Check sheet for the modelled part. Datum: model origin and axes. Units: mm. A direction names the side the tool comes from. Give positions to 0.01 mm unless a question says otherwise; leave off trailing zeros. Order: outer loops, then holes, each group sorted by start corner. A loop starts at its lowest first (then second) coordinate and runs counter-clockwise, first axis right, second up. Notation, with made-up numbers: (55.5, 34.5) - (95.5, 34.5) arc R29 cw to (95.5, 64.5) - close; hole circle Ø3 at (-30.5, 24.5). An arc over 180 degrees is marked (long way). Answer in a Markdown table with one row per item.
from build123d import *

# Parameters (mm, degrees)
F0_R     = 2.55
F1_DEPTH = 100
F2_R     = 2.75
F3_DEPTH = 15
F4_R     = 3


with BuildPart() as f1:
    # F0 (on Right) → F1 (new body)
    with BuildSketch(Plane.YZ):
        with BuildLine():
            Line((0, 57.5), (0, 0))
            Line((0, 0), (55, 0))
            Line((55, 0), (55, 15))
            Line((55, 15), (33, 15))
            ThreePointArc((33, 15), (27.343146, 17.343146), (25, 23))
            Line((25, 23), (25, 57.5))
            Line((25, 57.5), (0, 57.5))
        make_face()
        with Locations((12.5, 45)):
            Circle(F0_R, mode=Mode.SUBTRACT)
    extrude(amount=F1_DEPTH)

    # F2 (on Top) → F3 (cut)
    with BuildSketch(Plane.XY):
        with Locations((15, 45)):
            Circle(F2_R)
        with Locations((85, 45)):
            Circle(F2_R)
    extrude(amount=F3_DEPTH, mode=Mode.SUBTRACT)

    # F4
    f4_edges = [f1.edges().sort_by_distance(p)[0] for p in [
        (100, 12.5, 57.5),
        (0, 12.5, 57.5),
        (50, 25, 57.5),
        (50, 0, 57.5),
        (100, 44, 15),
        (50, 55, 15),
        (0, 44, 15),
        (100, 0, 28.75),
        (0, 0, 28.75),
        (0, 55, 7.5),
        (100, 55, 7.5),
    ]]
    fillet(f4_edges, radius=F4_R)


solid = f1.part
(1) Mould release check, pull along Z, two halves, no side actions. Record for faces 1 (the cylindrical face through (49.342, 27.406, 17.281)), 2 (the cylindrical face through (49.3, 10.6, 46.7)), 3 (the flat face through (49, 27, 0)): pulls with the +Z half, pulls with the -Z half, needs draft (parallel to the pull), parting line crosses it, or undercut.
Geometry says:
| item | result |
|---|---|
| face 1 | pulls with the +Z half |
| face 2 | undercut |
| face 3 | pulls with the -Z half |
(2) Access from +Z, -Z, +X, -X, +Y, -Y to the whole of each face (thin tool, end or side, straight path). Record for faces 4 (the cylindrical face through (0.86, 42.37, 14.1)), 5 (the flat face through (49, 43, 15)), 6 (the cylindrical face through (99.1, 0.86, 26.87)).
Geometry says:
| item | result |
|---|---|
| face 4 | +Z, -X, +Y |
| face 5 | +Z, +X, -X, +Y |
| face 6 | +Z, -Z, +X, -Y |
(3) Thickness scan on L1, parallel to Y at x = 85, z = 9.5; L2, parallel to Z at x = 58, y = 40.5; L3, parallel to Z at x = 34, y = 12.5. Record the ranges inside material, lowest first.
Geometry says:
| item | result |
|---|---|
| L1 | 0 to 42.25, 47.75 to 55 |
| L2 | 0 to 15 |
| L3 | 0 to 42.45, 47.55 to 57.5 |
(4) Cross-section at B-B, the plane x = 15. Record the cut outline in (y, z).
Geometry says:
| item | result |
|---|---|
| outline | (0, 0) - (42.25, 0) - (42.25, 15) - (33, 15) arc R8 cw to (25, 23) - (25, 54.5) arc R3 ccw to (22, 57.5) - (3, 57.5) arc R3 ccw to (0, 54.5) - close; (47.75, 0) - (55, 0) - (55, 12) arc R3 ccw to (52, 15) - (47.75, 15) - close; hole circle Ø5.1 at (12.5, 45) |
(5) Cross-section at A-A, the plane y = 12.5. Record the cut outline in (x, z).
Geometry says:
| item | result |
|---|---|
| outline | (0, 0) - (100, 0) - (100, 42.45) - (0, 42.45) - close; (0, 47.55) - (100, 47.55) - (100, 54.5) arc R3 ccw to (97, 57.5) - (3, 57.5) arc R3 ccw to (0, 54.5) - close |
(6) Cross-section at C-C, the plane z = 45. Record the cut outline in (x, y).
Geometry says:
| item | result |
|---|---|
| outline | (0, 3) arc R3 ccw to (3, 0) - (97, 0) arc R3 ccw to (100, 3) - (100, 9.95) - (0, 9.95) - close; (0, 15.05) - (100, 15.05) - (100, 22) arc R3 ccw to (97, 25) - (3, 25) arc R3 ccw to (0, 22) - close |
(7) Gauge pin test, flat ends, axial feed: P1, Ø9, axis at x = 15, y = 45, coming from the -Z side; P2, Ø25, axis at x = 58, z = 42, coming from the +Y side; P3, Ø15, axis at x = 60.5, y = 45.5, coming from the +Z side. Record the tip position at first contact, or that the pin passes through.
Geometry says:
| item | result |
|---|---|
| P1 | z = 0 |
| P2 | y = 25 |
| P3 | z = 15 |
(8) Cross-section at D-D, the plane y = 45. Record the cut outline in (x, z).
Geometry says:
| item | result |
|---|---|
| outline | (0, 0) - (12.25, 0) - (12.25, 15) - (3, 15) arc R3 ccw to (0, 12) - close; (17.75, 0) - (82.25, 0) - (82.25, 15) - (17.75, 15) - close; (87.75, 0) - (100, 0) - (100, 12) arc R3 ccw to (97, 15) - (87.75, 15) - close |
